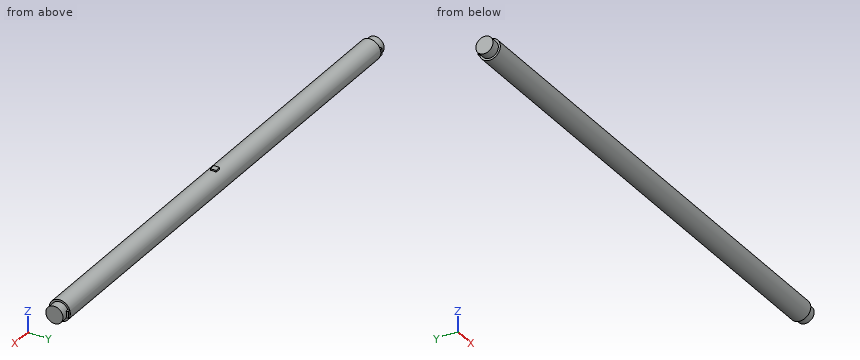
from build123d import *

# Parameters (mm, degrees)
BOSS_EXTRUDE1_REACH      = 994.465
BOSS_EXTRUDE1_END_RADIUS = 40
SKETCH4_W                = 22.36
SKETCH4_H                = 22
BOSS_EXTRUDE2_DEPTH      = 10


with BuildPart() as part:
    # Sketch1 → Revolve1 (revolve)
    with BuildSketch(Plane.XY):
        Polygon((-988, 0), (-988, 32.5), (-955, 32.5), (-955, 40), (955, 40), (955, 32.5), (988, 32.5), (988, 0), align=None)
    revolve(axis=Axis((988, 0, 0), (-1, 0, 0)))

    # Boss-Extrude1: up to this cylinder (the profile starts outside it)
    boss_extrude1_end = Plane(origin=(0, 0, 0), z_dir=(1, 0, 0)) * Cylinder(BOSS_EXTRUDE1_END_RADIUS, 2069.93, mode=Mode.PRIVATE)
    # Sketch4 → Boss-Extrude1 (add, up to the surface)
    with BuildSketch(Plane.XY.offset(45.1), mode=Mode.PRIVATE) as boss_extrude1_sk1:
        Rectangle(SKETCH4_W, SKETCH4_H)
    boss_extrude1_tool1 = extrude(boss_extrude1_sk1.sketch, amount=-BOSS_EXTRUDE1_REACH, mode=Mode.PRIVATE) - boss_extrude1_end
    add(boss_extrude1_tool1.solids().sort_by_distance((0, 0, 45.1))[0])

    # Sketch5 → Boss-Extrude2 (add)
    with BuildSketch(Plane.ZY.offset(955)):
        with BuildLine():
            Line((-12.5, 30), (-12.5, 39.13))
            Line((-12.5, 39.13), (12.5, 39.13))
            Line((12.5, 39.13), (12.5, 30))
            ThreePointArc((12.5, 30), (0, 32.5), (-12.5, 30))
        make_face()
    boss_extrude2 = extrude(amount=BOSS_EXTRUDE2_DEPTH)

    # Mirror1: Boss-Extrude2 across plane
    add(boss_extrude2.mirror(Plane.ZY))


solid = part.part
Source: CAD feature listing. Evaluate the final solid. Frame: model axes, mm. Round coordinates to 2 decimals unless told otherwise and drop trailing zeros. Order: outer loops, then holes, each group sorted by start corner. A loop starts at its lowest first (then second) coordinate and runs counter-clockwise, first axis right, second up. Notation, with made-up numbers: (-13.5, 8.5) - (30.5, 8.5) arc R19 ccw to (30.5, 19.5) - close; hole circle Ø8 at (-13.5, 53). An arc over 180 degrees is marked (long way). Use a Markdown table: item, result. Add a question column.
1. Line query: probe 1 along X at (y, z) = (6.5, 42); probe 2 along Z at (x, y) = (-573, -23.5); probe 3 along Z at (x, y) = (888.5, -2.5). Output: solid intervals per line, ascending.
2. Section query A-A (x = -644.5). Return the cut outline in (y, z), then the cut area to 3 significant figures.
3. First-contact query: pin 1 (6 mm diameter, centred on x = 721, y = -17.5, fed in from +Z); pin 2 (0.9 mm diameter, centred on y = 38.5, z = 10, fed in from -X); pin 3 (10 mm diameter, centred on x = -960.5, y = 33, fed in from +Z). Flat tips, straight axial feed; report the tip coordinate or a pass-through.
Derived:
| question | item | result |
|---|---|---|
| 1 | probe 1 | -11.18 to 11.18 |
| 1 | probe 2 | -32.37 to 32.37 |
| 1 | probe 3 | -39.92 to 39.92 |
| 2 | outline | circle Ø80 at (0, 0) |
| 2 | area | 5,030 mm2 |
| 3 | pin 1 | z = 37.28 |
| 3 | pin 2 | x = -965 |
| 3 | pin 3 | z = 16.5 |
